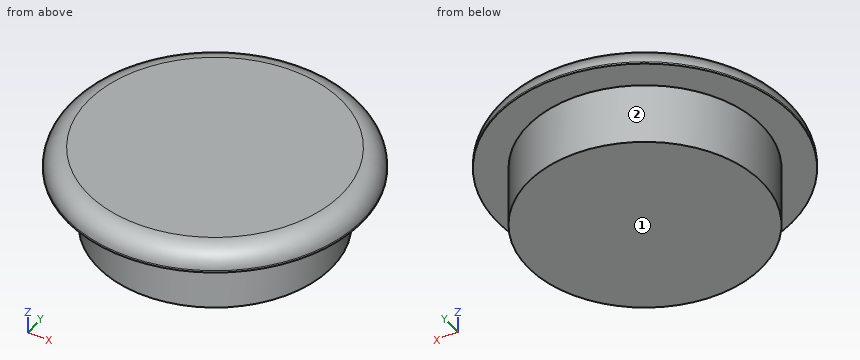
Autodesk Fusion 360 part; units mm, degrees
sketch "Sketch1" plane through (0, 0, 0) normal (0, 0, 1) x (1, 0, 0)
  circle A0 centre (0, 0) radius 11.5
  circle A1 centre (0, 0) radius 14.5
  dimension "d1" = 23
  dimension "d2" = 29
extrude "Extrude1" add sketch "Sketch1" along normal blind 2.2 contours A0 | A1
extrude "Extrude2" add sketch "Sketch1" against normal blind 6 contours A0
fillet "Fillet1" radius 2 1 edges at (-13.5187, -5.2434, 2.2)
Source: CAD feature listing. Evaluate the final solid. Frame: model axes, mm. Face numbers are marked on the shaded views. A direction names the side the tool comes from. Give positions to 0.01 mm unless a question says otherwise; leave off trailing zeros. Write each loop counter-clockwise with the first axis right and the second up, starting at its lowest first coordinate (ties: lowest second). Pieces come first, ordered by that corner, then holes. Notation, with made-up numbers: M 1,26.5 L 36,26.5 A15 cw 36,53.5 Z; hole C 16.25,59 d9. An arc over 180 degrees is marked long. Return JSON: item names as keys, results as strings. Group by question number.
1) Cut plane C-C, the plane z = -3.75. Output: boundary loops of the cut face in (x, y).
2) Set-up query: the marked faces 1 and 2. Return all of +Z, -Z, +X, -X, +Y, -Y with unobstructed straight access to the full face (end or side cutting, diameter ignored); none if empty.
3) Ray query, L1, parallel to Z at x = -10.5, y = 6.25; L2, parallel to Y at x = 0, z = -5; L3, parallel to Y at x = 1.5, z = 0.25. Return the intervals inside material, ascending.
4) First-contact query: pin 1 Ø3 at (y, z) = (-7.5, -1) entering from -X; pin 2 Ø1.5 at (x, y) = (-9.5, 9.5) entering from +Z; pin 3 Ø3 at (x, z) = (5, -0.5) entering from -Y. Flat tips, straight axial feed; report the tip coordinate or a pass-through.
5) Cut plane A-A, the plane y = 0. Output: boundary loops of the cut face in (x, z), then the cut area to 3 significant figures.
Data:
{
 "1": {"outline": "C 0,0 d23"},
 "2": {"face 1": "-Z, +X, -X, +Y, -Y", "face 2": "-Z"},
 "3": {"L1": "z = 0 to 2.2", "L2": "y = -11.5 to 11.5", "L3": "y = -14.42 to 14.42"},
 "4": {"pin 1": "stops at x = -13.02", "pin 2": "stops at z = 2.19", "pin 3": "stops at y = -14.05"},
 "5": {"outline": "M -14.5,0 L -11.5,0 L -11.5,-6 L 11.5,-6 L 11.5,0 L 14.5,0 L 14.5,0.2 A2 ccw 12.5,2.2 L -12.5,2.2 A2 ccw -14.5,0.2 Z", "area": "200 mm²"}
}
